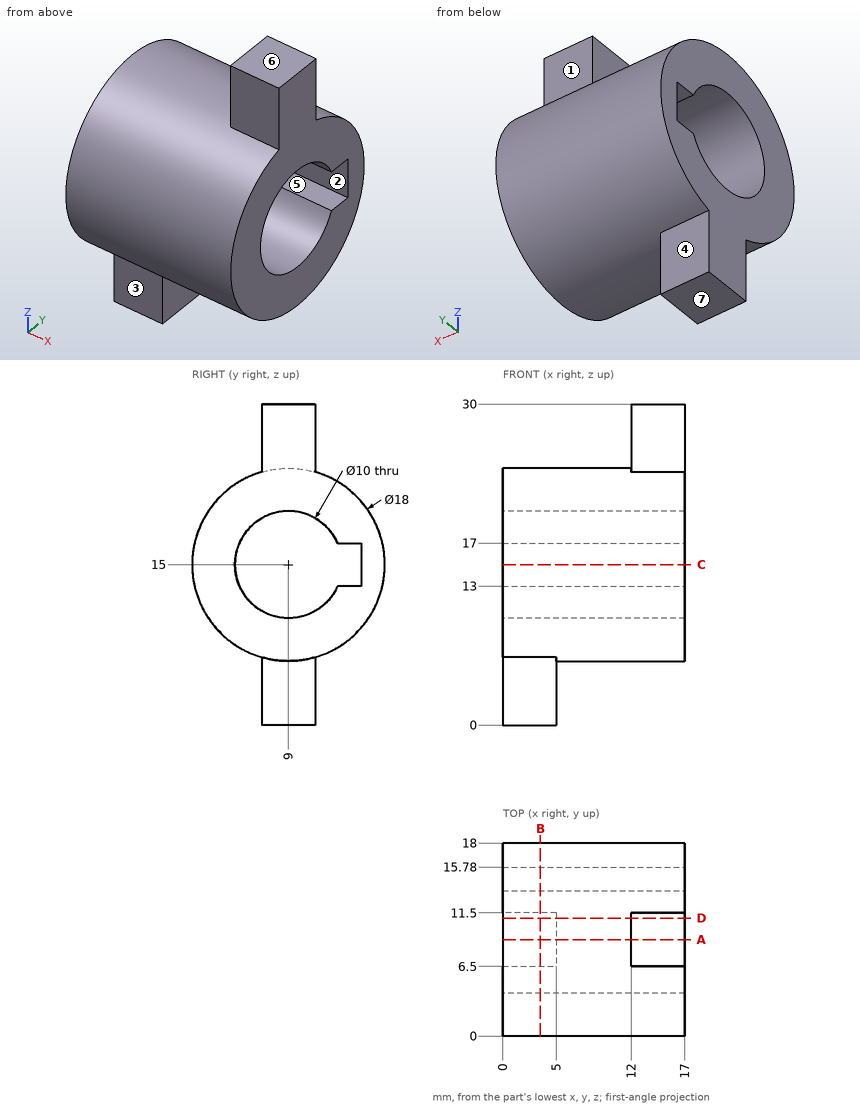
Could you check a few things on this drawing? It's one solid part, dimensions in mm from its lowest x, y, z. A direction names the side the tool comes from. Round coordinates to 2 decimals unless told otherwise and drop trailing zeros. Order: outer loops, then holes, each group sorted by start corner. A loop starts at its lowest first (then second) coordinate and runs counter-clockwise, first axis right, second up.
(1) Imagine slicing it at B-B (x = 3.5). Write out the boundary of the cut face in (y, z), plus the area to 3 significant figures.
Response values:
outline: (6.5, 0) - (11.5, 0) - (11.5, 6.35) arc R9 ccw (long way) to (6.5, 6.35) - close; hole (13.58, 13) - (15.78, 13) - (15.78, 17) - (13.58, 17) arc R5 ccw (long way) to start
area: 199 mm2
(2) If we mould it in two halves opening along Z, with no side actions, what happens to the marked faces 5, 6 and 7? For each: released by +Z, released by -Z, zero draft, split by the parting line, or undercut.
Response values:
face 5: undercut
face 6: released by +Z
face 7: released by -Z
(3) Imagine slicing it at C-C (z = 15). Write out the boundary of the cut face in (x, y).
Response values:
outline: (0, 0) - (17, 0) - (17, 4) - (0, 4) - close; (0, 15.78) - (17, 15.78) - (17, 18) - (0, 18) - close
(4) I'm going to push flat-ended pins straight in: pin 1 (5 mm diameter, centred on x = 11, z = 21, fed in from -Y); pin 2 (1.1 mm diameter, centred on x = 6, y = 14.5, fed in from +Z); pin 3 (1.5 mm diameter, centred on y = 10, z = 3.5, fed in from +X); pin 4 (8 mm diameter, centred on y = 9, z = 15, fed in from -X). Where does each tip first touch, or does it pass through?
Response values:
pin 1: stops at y = 0.71
pin 2: stops at z = 22.52
pin 3: stops at x = 5
pin 4: passes through
(5) Please list where these lines run through material, in increasing order: line 1 along Y through (x, z) = (13.25, 15); line 2 along Z through (x, y) = (5.5, 9); line 3 along Y through (x, z) = (0.75, 5.75).
Response values:
line 1: y = 0 to 4, 15.78 to 18
line 2: z = 6 to 10, 20 to 24
line 3: y = 6.5 to 11.5
(6) Which directions (+Z, -Z, +X, -X, +Y, -Y) give clear straight access to the entire face, cutting with the end or side of a thin tool? Please do the marked faces 1, 2, 3 and 4.
Response values:
face 1: +Z, +X, -X, +Y
face 2: +X, -X
face 3: -Z, +X, -X, -Y
face 4: -Z, +X, -X, +Y
(7) Imagine slicing it at D-D (y = 11). Write out the boundary of the cut face in (x, z).
Response values:
outline: (0, 0) - (5, 0) - (5, 6.23) - (17, 6.23) - (17, 10.42) - (0, 10.42) - close; (0, 19.58) - (17, 19.58) - (17, 30) - (12, 30) - (12, 23.77) - (0, 23.77) - close
(8) Imagine slicing it at A-A (y = 9). Write out the boundary of the cut face in (x, z).
Response values:
outline: (0, 0) - (5, 0) - (5, 6) - (17, 6) - (17, 10) - (0, 10) - close; (0, 20) - (17, 20) - (17, 30) - (12, 30) - (12, 24) - (0, 24) - close
